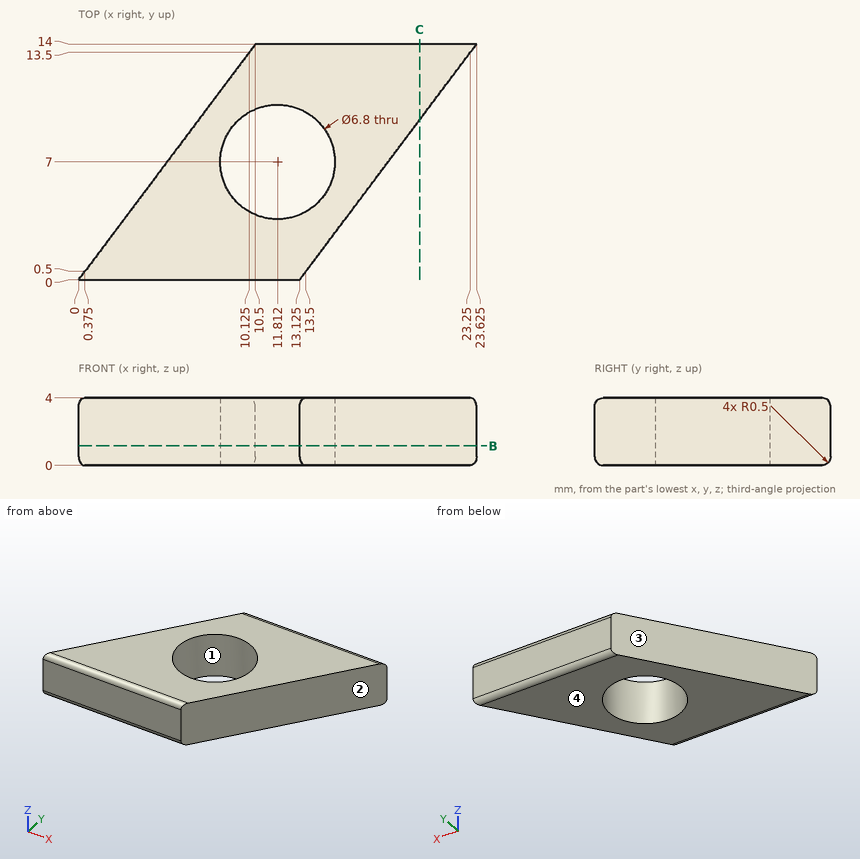
Study the drawing (mm; zero at the part's minimum x, y, z) and answer. Coordinates: 2 decimals unless noted, no trailing zeros. Write each loop counter-clockwise with the first axis right and the second up, starting at its lowest first coordinate (ties: lowest second). Pieces come first, ordered by that corner, then holes. Notation, with made-up numbers: (30, 31.25) - (59, 31.25) arc R27 ccw to (59, 61.25) - close; hole circle Ø5 at (21.5, 0). An arc over 180 degrees is marked (long way). Put each result on its own line as item: value.
1. Find the intervals of material crossed by line 1 along Y through (x, z) = (13.25, 0.85) (1 decimal); line 2 along Y through (x, z) = (12.5, 2); line 3 along Y through (x, z) = (3, 0.65), in increasing order. Write a range as from..to.
Answer sheet:
line 1: y = 0.2..3.9, 10.1..14
line 2: y = 0..3.67, 10.33..14
line 3: y = 0..4
2. Flat-ended cylindrical pins translate along their axes: pin 1 Ø2 at (y, z) = (9.5, 3.5) entering from +X; pin 2 Ø2 at (x, y) = (5, 10) entering from +Z. Find the tip coordinate at first contact, or state that the pin passes through.
Answer sheet:
pin 1: stops at x = 21
pin 2: passes through
3. The part is cut by section B-B on z = 1.15. Give the vertices of the cut face in (x, y) (1 decimal).
Answer sheet:
outline: (0, 0) - (13.1, 0) - (23.6, 14) - (10.5, 14) - close; hole circle Ø6.8 at (11.8, 7)
4. The part is cut by section C-C on x = 20.25. Give the vertices of the cut face in (y, z), plus the area to 3 significant figures.
Answer sheet:
outline: (9.5, 0) - (13.5, 0) arc R0.5 ccw to (14, 0.5) - (14, 3.5) arc R0.5 ccw to (13.5, 4) - (9.5, 4) - close
area: 17.9 mm^2
5. Determine the mould class of the marked faces 1, 2, 3 and 4 for opening direction X: pulls with the +X half, pulls with the -X half, needs draft (parallel to the pull), parting line crosses it, or undercut.
Answer sheet:
face 1: undercut
face 2: pulls with the +X half
face 3: pulls with the -X half
face 4: needs draft
